from build123d import *

# Parameters (mm, degrees)
F0_W     = 57.15
F0_H     = 31.75
F1_DEPTH = 38.1
F4_DEPTH = 177.8
F5_DEPTH = 12.7
F6_DEPTH = 12.7


with BuildPart() as f1:
    # F0 (on Front) → F1 (new body)
    with BuildSketch(Plane.XZ):
        with Locations((28.575, 15.875)):
            Rectangle(F0_W, F0_H)
    extrude(amount=F1_DEPTH)

    # F3 (on face) → F4 (cut)
    with BuildSketch(Plane.XZ.offset(38.1)):
        Polygon((57.15, 31.75), (44.541387, 31.75), (57.15, 0), align=None)
    extrude(amount=-F4_DEPTH, mode=Mode.SUBTRACT)

    # F3 (on face) → F5 (cut)
    with BuildSketch(Plane.XZ.offset(38.1)):
        Polygon((44.541387, 31.75), (19.141387, 31.75), (31.737559, 0), (57.137559, 0), (57.15, 0), align=None)
    extrude(amount=-F5_DEPTH, mode=Mode.SUBTRACT)

    # F2 (on face) → F6 (cut)
    with BuildSketch(Plane(origin=(0, 0, 0), x_dir=(-1, 0, 0), z_dir=(0, 1, 0))):
        Polygon((-31.75, 0), (-19.05, 31.75), (-57.15, 31.75), (-57.15, 0), align=None)
    extrude(amount=-F6_DEPTH, mode=Mode.SUBTRACT)


solid = f1.part
Design review of the part built by this model. Coordinates are the model's own, in mm. A direction names the side the tool comes from. Coordinates: 2 decimals unless noted, no trailing zeros. Write each loop counter-clockwise with the first axis right and the second up, starting at its lowest first coordinate (ties: lowest second). Pieces come first, ordered by that corner, then holes. Notation, with made-up numbers: (-19, -39) - (12, -39) arc R10 ccw to (12, -22) - close; hole circle Ø4 at (-1.5, -34.75). An arc over 180 degrees is marked (long way). Use one line per item in the form item = value.
Q1. Insertion check: pin 1 Ø4 at (x, z) = (39, 9.5) entering from -Y. The pin has a flat end and moves straight along its axis. Give the tip position at first contact, or say it passes through.
Taken from the geometry:
pin_1 = -25.4
Q2. Consider section A-A (z = 9). Write out the cut boundary in (x, y).
Taken from the geometry:
outline = (0, -38.1) - (28.17, -38.1) - (28.17, -25.4) - (53.58, -25.4) - (53.58, -12.7) - (28.15, -12.7) - (28.15, 0) - (0, 0) - close
Q3. Consider section D-D (y = -2.5). Write out the cut boundary in (x, z), plus the area to 3 significant figures.
Taken from the geometry:
outline = (0, 0) - (31.75, 0) - (19.05, 31.75) - (0, 31.75) - close
area = 806 mm^2
Q4. For probe 1 along Y at (x, z) = (46, 5.5); probe 2 along X at (y, z) = (-15, 2); probe 3 along X at (y, z) = (-16, 17), list the stretches that pass through material, from the lowest coordinate up.
Taken from the geometry:
probe_1 = -25.4 to -12.7
probe_2 = 0 to 56.36
probe_3 = 0 to 50.4
Q5. Consider section B-B (x = 20). Write out the cut boundary in (y, z) (3 decimals), plus the area to 3 significant figures.
Taken from the geometry:
outline = (-38.1, 0) - (0, 0) - (0, 29.375) - (-12.7, 29.375) - (-12.7, 31.75) - (-25.4, 31.75) - (-25.4, 29.586) - (-38.1, 29.586) - close
area = 1,150 mm^2
Q6. Machinability: for faces 1 (the flat face through (25.49, -6.26, 15.65)), 2 (the flat face through (25.35, -31.84, 16.1)), 3 (the flat face through (12, 0, 16)), which of the approach directions +Z, -Z, +X, -X, +Y, -Y give a long, thin tool a straight path to every point of the face, cutting with its end or side? Answer none if there is none.
Taken from the geometry:
face_1 = +Z, +X, +Y
face_2 = +Z, +X, -Y
face_3 = +Z, -Z, +X, -X, +Y
Q7. Consider section C-C (y = -32). Write out the cut boundary in (x, z), plus the area to 3 significant figures.
Taken from the geometry:
outline = (0, 0) - (31.74, 0) - (19.14, 31.75) - (0, 31.75) - close
area = 808 mm^2
